CAD build for the part. Positions are in the model's coordinates, mm. A direction names the side the tool comes from. Give positions to 0.01 mm unless a question says otherwise; leave off trailing zeros. Order: outer loops, then holes, each group sorted by start corner. A loop starts at its lowest first (then second) coordinate and runs counter-clockwise, first axis right, second up. Notation, with made-up numbers: (54, 48) -> (85, 48) arc R9 cw to (85, 54) -> close; hole circle Ø4 at (21, 34). An arc over 180 degrees is marked (long way). Answer as CSV lines item,"result".
```python
from build123d import *

# Parameters (mm, degrees)
BOSS_EXTRUDE1_DEPTH = 12.7
CUT_EXTRUDE1_DEPTH  = 155.131437711
CUT_EXTRUDE2_REACH  = 110.694
FILLET1_R           = 1.5875


with BuildPart() as part:
    # Sketch1 → Boss-Extrude1 (new body)
    with BuildSketch(Plane(origin=(0, 0, 0), x_dir=(0, 0, -1), z_dir=(1, 0, 0))):
        Polygon((-95.25, 0), (95.25, 0), (77.47, 48.850148518), (77.47, 12.7), (39.37, 12.7), (39.37, 50.8), (-44.45, 50.8), align=None)
    extrude(amount=BOSS_EXTRUDE1_DEPTH)

    # Sketch2 → Cut-Extrude1 (cut, through all, along a direction that is not the sketch's normal)
    with BuildSketch(Plane(origin=(0, 0, 0), x_dir=(-1, 0, 0), z_dir=(0, -1, 0))):
        Polygon((0, -95.25), (-12.7, -95.25), (-12.7, -87.63), align=None)
    extrude(amount=-CUT_EXTRUDE1_DEPTH, dir=(0, -0.7071067811865438, 0.7071067811865512), mode=Mode.SUBTRACT)

    # Sketch4 → Cut-Extrude2 (cut, up to next)
    with BuildSketch(Plane(origin=(12.7, 0, 0), x_dir=(0, 0, -1), z_dir=(1, 0, 0)), mode=Mode.PRIVATE) as cut_extrude2_sk1:
        Polygon((-56.969487758, 12.7), (-28.394487758, 41.275), (-28.394487758, 12.7), align=None)
    cut_extrude2_tool1 = extrude(cut_extrude2_sk1.sketch, amount=-CUT_EXTRUDE2_REACH, mode=Mode.PRIVATE) & part.part
    # Sketch4 → Cut-Extrude2 (cut, up to next)
    with BuildSketch(Plane(origin=(12.7, 0, 0), x_dir=(0, 0, -1), z_dir=(1, 0, 0)), mode=Mode.PRIVATE) as cut_extrude2_sk2:
        Polygon((-15.694487758, 12.7), (-15.694487758, 41.275), (12.880512242, 12.7), align=None)
    cut_extrude2_tool2 = extrude(cut_extrude2_sk2.sketch, amount=-CUT_EXTRUDE2_REACH, mode=Mode.PRIVATE) & part.part
    # Sketch4 → Cut-Extrude2 (cut, up to next)
    with BuildSketch(Plane(origin=(12.7, 0, 0), x_dir=(0, 0, -1), z_dir=(1, 0, 0)), mode=Mode.PRIVATE) as cut_extrude2_sk3:
        Polygon((2.266024484, 41.275), (26.67, 16.871024484), (26.67, 41.275), align=None)
    cut_extrude2_tool3 = extrude(cut_extrude2_sk3.sketch, amount=-CUT_EXTRUDE2_REACH, mode=Mode.PRIVATE) & part.part
    add(cut_extrude2_tool1.solids().sort_by_distance((12.7, 22.225, 37.919488))[0], mode=Mode.SUBTRACT)
    add(cut_extrude2_tool2.solids().sort_by_distance((12.7, 22.225, 6.169488))[0], mode=Mode.SUBTRACT)
    add(cut_extrude2_tool3.solids().sort_by_distance((12.7, 33.140341, -18.535341))[0], mode=Mode.SUBTRACT)

    # Fillet1
    fillet1_edges = [part.edges().sort_by_distance(p)[0] for p in [
        (6.35, 12.7, 28.394487758),
        (6.35, 12.7, 56.969487758),
        (6.35, 41.275, 28.394487758),
        (6.35, 41.275, -2.266024484),
        (6.35, 41.275, -26.67),
        (6.35, 16.871024484, -26.67),
        (6.35, 12.7, -12.880512242),
        (6.35, 12.7, 15.694487758),
        (6.35, 41.275, 15.694487758),
    ]]
    fillet(fillet1_edges, radius=FILLET1_R)


solid = part.part
```
1) Pin check, flat tips, straight feed: P1, Ø8, axis at y = 16, z = 71.5, coming from the -X side; P2, Ø4, axis at x = 6, y = 37.5, coming from the -Z side; P3, Ø6.5, axis at x = 3.5, y = 27.5, coming from the +Z side; P4, Ø4, axis at x = 8.5, y = 27.5, coming from the +Z side. Stop position of each tip, or through.
Data:
P1,"stops at x = 0"
P2,"stops at z = -82.33"
P3,"stops at z = 69.44"
P4,"stops at z = 64.98"
2) Band-saw the part on B-B, the plane y = 45. Write the cut outline in (x, z).
Data:
outline,"(0, -78.87) -> (12.7, -78.87) -> (12.7, -77.47) -> (0, -77.47) -> close; (0, -39.37) -> (12.7, -39.37) -> (12.7, 42.63) -> (0, 50.25) -> close"
3) Wall check: line 1 along Z through (x, y) = (7.25, 39.5); line 2 along Z through (x, y) = (2.5, 20.5); line 3 along Z through (x, y) = (8, 28). Give the ranges that are in metal, low to high. Write a range as [from, to].
Data:
line 1,"z = [-80.87, -77.47], [-39.37, -26.67], [-4.52, 51.4]"
line 2,"z = [-87.79, -77.47], [-39.37, -26.66], [-23.04, -5.08], [15.69, 28.39], [49.17, 73.25]"
line 3,"z = [-85.06, -77.47], [-39.37, -26.67], [-15.54, 2.42], [15.69, 28.39], [41.67, 62.45]"
4) Which spindle directions (+Z, -Z, +X, -X, +Y, -Y) get a long thin tool onto all of the face, cutting with end or side? Do faces 4 (the flat face through (6, 12.7, -59)), 5 (the flat face through (6.261, 24.083, -86.484)), 6 (the flat face through (6, 30, -26.67)). Say none if no direction does.
Data:
face 4,"+X, -X, +Y"
face 5,"-Z, +X, -X, +Y"
face 6,"+X, -X"
5) Band-saw the part on C-C, the plane z = -1.5. Write the cut outline in (x, y).
Data:
outline,"(0, 0) -> (12.7, 0) -> (12.7, 12.7) -> (0, 12.7) -> close; (0, 24.08) -> (12.7, 24.08) -> (12.7, 50.8) -> (0, 50.8) -> close"
6) Pull direction Y, two halves, no side cores. Call faces 1 (the flat face through (6.753, 25.044, 66.154)), 2 (the flat face through (6, 0, 1)), 3 (the flat face through (6.439, 29.206, -14.335)): pulls with the +Y half, pulls with the -Y half, needs draft (parallel to the pull), parting line crosses it, or undercut.
Data:
face 1,"pulls with the +Y half"
face 2,"pulls with the -Y half"
face 3,"undercut"
7) Band-saw the part on D-D, the plane y = 32.5. Write the cut outline in (x, z).
Data:
outline,"(0, -83.42) -> (12.7, -83.42) -> (12.7, -77.47) -> (0, -77.47) -> close; (0, -39.37) -> (12.7, -39.37) -> (12.7, -26.67) -> (0, -26.67) -> close; (0, -11.04) -> (12.7, -11.04) -> (12.7, 6.92) -> (0, 6.92) -> close; (0, 15.69) -> (12.7, 15.69) -> (12.7, 28.39) -> (0, 28.39) -> close; (0, 37.17) -> (12.7, 37.17) -> (12.7, 55.13) -> (0, 62.75) -> close"
8) Band-saw the part on A-A, the plane x = 2. Give the number of separate pieces and of enclosed holes in the cut face, then the cut area to 3 significant figures.
Data:
separate pieces,"1"
enclosed holes,"3"
area,"5,310 mm2"
